CAD build for the part. Positions are in the model's coordinates, mm. Face numbers are marked on the shaded views. Coordinates: 2 decimals unless noted, no trailing zeros. Write each loop counter-clockwise with the first axis right and the second up, starting at its lowest first coordinate (ties: lowest second). Pieces come first, ordered by that corner, then holes. Notation, with made-up numbers: (11, -19.5) - (21, -19.5) arc R34 cw to (21, 16.5) - close; hole circle Ø3 at (-39, 22.25). An arc over 180 degrees is marked (long way). Answer in a Markdown table with one row per item. Add a question column.
Q1. Two-plate mould, pull along Z, no slides. Class the marked faces 1 and 2: +Z half, -Z half, draft (parallel to the pull), parting line (faces both ways), or undercut.
Q2. Pin check, flat tips, straight feed: pin 1 (8 mm diameter, centred on x = 1, y = -12, fed in from +Z); pin 2 (10 mm diameter, centred on x = 1.5, z = -163, fed in from -Y); pin 3 (4 mm diameter, centred on x = -4.5, y = 13.5, fed in from +Z); pin 4 (3 mm diameter, centred on x = 5.5, z = -173.5, fed in from -Y). Stop position of each tip, or through.
Q3. Drill centre lines: line 1 along Y through (x, z) = (-1, -328); line 2 along X through (y, z) = (1, -310.5); line 3 along Z through (x, y) = (5, 17.5). Where is each one in solid material? Low to high. Write a range as from..to.
Q4. Band-saw the part on A-A (z = -149.5). List the corners of the cut face in (x, y), and give its area (3 significant figures).
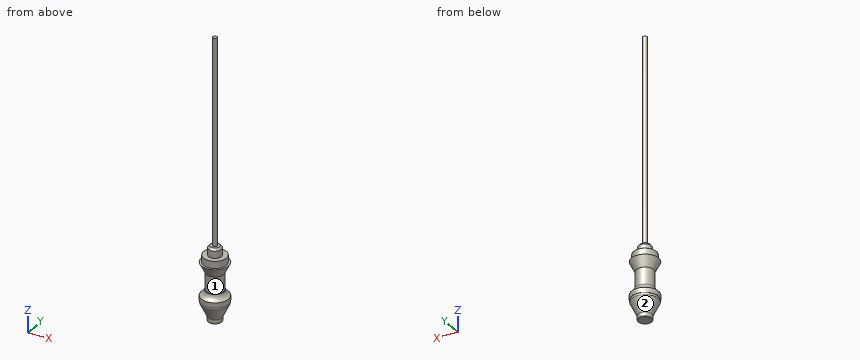
```python
from build123d import *


with BuildPart() as part:
    # Эскиз1 → Повернуть1 (revolve)
    with BuildSketch(Plane(origin=(0, 0, 0), x_dir=(0, 0, -1), z_dir=(1, 0, 0)), mode=Mode.PRIVATE) as revolve_1_sk:
        with BuildLine():
            Line((0, 0), (0, 3))
            Line((0, 3), (289, 3))
            Line((289, 3), (289, 6.5))
            Line((289, 6.5), (291.999073931, 9))
            Line((291.999073931, 9), (301.999073931, 9))
            Line((301.999073931, 9), (301.999073931, 16))
            Line((301.999073931, 16), (311.999073931, 16))
            Line((311.999073931, 16), (311.999073931, 19))
            Line((311.999073931, 19), (325.999073931, 12))
            Line((325.999073931, 12), (349.999073931, 12))
            Line((349.999073931, 12), (349.999073931, 12.7))
            ThreePointArc((349.999073931, 12.7), (354.861013139, 14.755474022), (357.999073931, 19))
            Line((357.999073931, 19), (365, 19))
            Line((365, 19), (365, 18.5))
            Line((365, 18.5), (368, 18.5))
            Line((368, 18.5), (387, 9.5))
            Line((387, 9.5), (392.2, 9.5))
            ThreePointArc((392.2, 9.5), (392.765685425, 9.265685425), (393, 8.7))
            Line((393, 8.7), (393, 0))
            Line((393, 0), (0, 0))
        make_face()
    revolve(revolve_1_sk.sketch.rotate(Axis((0, 0, 0), (0, 0, -1)), 90), axis=Axis((0, 0, 0), (0, 0, -1)))


solid = part.part
```
Checked values:
| question | item | result |
|---|---|---|
| 1 | face 1 | undercut |
| 1 | face 2 | -Z half |
| 2 | pin 1 | stops at z = -290.85 |
| 2 | pin 2 | stops at y = -3 |
| 2 | pin 3 | stops at z = -302 |
| 2 | pin 4 | passes through |
| 3 | line 1 | y = -11.96..11.96 |
| 3 | line 2 | x = -15.97..15.97 |
| 3 | line 3 | z = -368.63..-357.65, -313.6..-312 |
| 4 | outline | circle Ø6 at (0, 0) |
| 4 | area | 28.3 mm² |
